```python
from build123d import *

# Parameters (mm, degrees)
SKETCH022_R           = 4.75
SKETCH022_R_2         = 2.25
PAD011_DEPTH          = 1.55
SKETCH023_W           = 4.7
SKETCH023_H           = 2
PAD012_DEPTH          = 1.55
SKETCH025_W           = 1.2
SKETCH025_H           = 0.7
PAD013_DEPTH          = 0.65
POLARPATTERN003_COUNT = 4
SKETCH024_R           = 4.75
SKETCH024_R_2         = 2.75
POCKET009_DEPTH       = 0.775


with BuildPart() as part:
    # Sketch022 → Pad011 (new body)
    with BuildSketch(Plane.XY):
        Circle(SKETCH022_R)
        Circle(SKETCH022_R_2, mode=Mode.SUBTRACT)
    extrude(amount=-PAD011_DEPTH)

    # Sketch023 → Pad012 (join)
    with BuildSketch(Plane.XY):
        with Locations((0, -4.5)):
            Rectangle(SKETCH023_W, SKETCH023_H)
    pad012 = extrude(amount=-PAD012_DEPTH)

    # Sketch025 → Pad013 (join)
    with BuildSketch(Plane.XY.offset(-1.55)):
        with Locations((0, -5.85)):
            Rectangle(SKETCH025_W, SKETCH025_H)
    pad013 = extrude(amount=PAD013_DEPTH)

    # PolarPattern003: Pad012, Pad013 ×4 about axis
    polarpattern003_axis = Axis((0, 0, 0), (0, 0, 1))
    for i in range(1, POLARPATTERN003_COUNT):
        add(pad012.rotate(polarpattern003_axis, i * 360 / POLARPATTERN003_COUNT))
        add(pad013.rotate(polarpattern003_axis, i * 360 / POLARPATTERN003_COUNT))

    # Sketch024 → Pocket009 (cut)
    with BuildSketch(Plane.XY.offset(-1.55)):
        Circle(SKETCH024_R)
        Circle(SKETCH024_R_2, mode=Mode.SUBTRACT)
    extrude(amount=POCKET009_DEPTH, mode=Mode.SUBTRACT)


with BuildPart() as part_1:
    # Body002 placement: moved
    add(part.part.moved(Location((0, 0, -1))))


solid = part_1.part
```
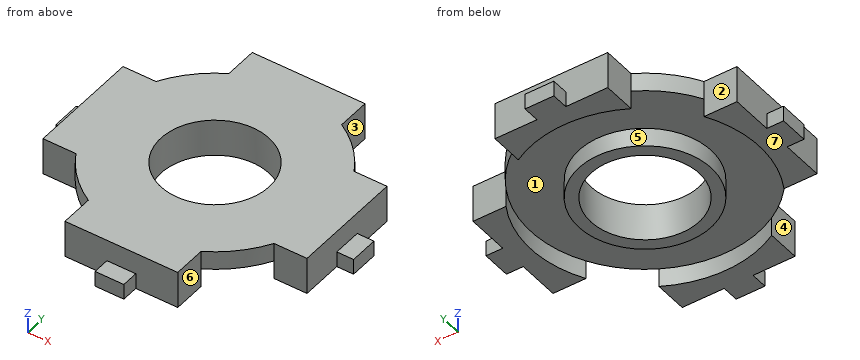
Read the model definition and answer for the solid it produces. Units are mm, in the model's axes. Face numbers are marked on the shaded views. A direction names the side the tool comes from. Give positions to 0.01 mm unless a question says otherwise; leave off trailing zeros. Loops run counter-clockwise (first coordinate to the right, second up) from the corner with the lowest first, then second, coordinate; pieces in that order, holes last.
Item 1: Find the intervals of material crossed by line 1 along Y through (x, z) = (0, -2); line 2 along Y through (x, z) = (-1, -2.2); line 3 along Y through (x, z) = (0, -1.25), in increasing order.
Item 2: For the marked faces 1, 2, 3 and 4, determine the directions among +Z, -Z, +X, -X, +Y, -Y from which every point of the face is accessible in a straight line to the end or side of a thin tool.
Item 3: The part is cut by section B-B (x = 0). Write down the section's boundary in (y, z) (3 decimals), and give its area (4 significant figures).
Item 4: The part is cut by section A-A (z = -2.3). Give the number of separate pieces and of enclosed holes in the cut face, and give its area (3 significant figures).
Item 5: Each of these flat-tipped pins is pushed along its axis until it touches: pin 1 Ø0.7 at (y, z) = (5, -2) entering from +X; pin 2 Ø0.7 at (x, z) = (6, -2) entering from -Y; pin 3 Ø0.5 at (x, z) = (1, -2) entering from -Y. Where does it stop, or does it pass through?
Item 6: The mould has two halves that part along X. Classify the marked faces 5, 6 and 7: released by +X, released by -X, zero draft, split by the parting line, or undercut.
Item 7: The part is cut by section D-D (z = -1.6). Write down the section's boundary in (x, y), and give its area (3 significant figures).
Taken from the geometry:
1. line 1: y = -6.2 to -4.75, -2.75 to -2.25, 2.25 to 2.75, 4.75 to 6.2
1. line 2: y = -5.5 to -4.64, -2.56 to -2.02, 2.02 to 2.56, 4.64 to 5.5
1. line 3: y = -5.5 to -2.25, 2.25 to 5.5
2. face 1: -Z
2. face 2: +Z, -Z, -X, +Y
2. face 3: +Z, -Z, +X, +Y
2. face 4: +Z, -Z, -X, -Y
3. outline: (-6.2, -2.55) - (-4.75, -2.55) - (-4.75, -1.775) - (-2.75, -1.775) - (-2.75, -2.55) - (-2.25, -2.55) - (-2.25, -1) - (-5.5, -1) - (-5.5, -1.9) - (-6.2, -1.9) - close; (2.25, -2.55) - (2.75, -2.55) - (2.75, -1.775) - (4.75, -1.775) - (4.75, -2.55) - (6.2, -2.55) - (6.2, -1.9) - (5.5, -1.9) - (5.5, -1) - (2.25, -1) - close
3. area: 7.885 mm2
4. separate pieces: 5
4. enclosed holes: 1
4. area: 29.1 mm2
5. pin 1: stops at x = 2.35
5. pin 2: stops at y = -0.6
5. pin 3: stops at y = -5.5
6. face 5: undercut
6. face 6: released by +X
6. face 7: zero draft
7. outline: (-5.5, -2.35) - (-4.13, -2.35) arc R4.75 ccw to (-2.35, -4.13) - (-2.35, -5.5) - (2.35, -5.5) - (2.35, -4.13) arc R4.75 ccw to (4.13, -2.35) - (5.5, -2.35) - (5.5, 2.35) - (4.13, 2.35) arc R4.75 ccw to (2.35, 4.13) - (2.35, 5.5) - (-2.35, 5.5) - (-2.35, 4.13) arc R4.75 ccw to (-4.13, 2.35) - (-5.5, 2.35) - close; hole circle Ø4.5 at (0, 0)
7. area: 72.9 mm2
